```python
from build123d import *

# Parameters (mm, degrees)
F1_DEPTH = 325
F2_W     = 250
F2_H     = 650
F3_DEPTH = 900


with BuildPart() as f1:
    # F0 (on Right) → F1 (new body, symmetric)
    with BuildSketch(Plane.YZ):
        Polygon((100, 875.2594227621), (650.2305358614, 489.9838537988), (722.4783731793, 544.4265042209), (214.6667939321, 900), (100, 900), align=None)
        Polygon((650.2305358614, 489.9838537988), (0, 0), (150, 0), (727.9826985434, 435.5412033767), align=None)
        Polygon((722.4783731793, 544.4265042209), (650.2305358614, 489.9838537988), (727.9826985434, 435.5412033767), (800.2305358614, 489.9838537988), align=None)
        Polygon((1194.3403394584, 900), (722.4783731793, 544.4265042209), (800.2305358614, 489.9838537988), (1250, 828.9094551131), (1250, 900), align=None)
        Polygon((800.2305358614, 489.9838537988), (727.9826985434, 435.5412033767), (1350, 0), (1500, 0), align=None)
    extrude(amount=F1_DEPTH, both=True)

    # F2 (on Top) → F3 (cut, through all)
    with BuildSketch(Plane.XY):
        with Locations((200, 675)):
            Rectangle(F2_W, F2_H)
        with Locations((-200, 675)):
            Rectangle(F2_W, F2_H)
    extrude(amount=F3_DEPTH, mode=Mode.SUBTRACT)


solid = f1.part
```
CAD build for the part. Positions are in the model's coordinates, mm. A direction names the side the tool comes from. Coordinates: 2 decimals unless noted, no trailing zeros. Order: outer loops, then holes, each group sorted by start corner. A loop starts at its lowest first (then second) coordinate and runs counter-clockwise, first axis right, second up.
(1) Drill centre lines: L1, parallel to X at y = 965.5, z = 358.5; L2, parallel to Y at x = -25.5, z = 774; L3, parallel to Y at x = -10, z = 629.5. Where is each one in solid material? Low to high.
Solution:
L1: x = -75 to 75
L2: y = 244.61 to 394.61, 1027.13 to 1177.13
L3: y = 450.98 to 600.98, 835.37 to 985.37
(2) Pin check, flat tips, straight feed: pin 1 Ø1 at (x, z) = (-29, 332) entering from -Y; pin 2 Ø5 at (x, z) = (-88, 333) entering from -Y; pin 3 Ø1 at (x, z) = (88.5, 715.5) entering from +Y. Stop position of each tip, or through.
Solution:
pin 1: stops at y = 439.92
pin 2: stops at y = 1000
pin 3: stops at y = 1100.16
(3) Saw through at A-A, the plane x = -121. Write the cut outline in (y, z), and give its area (3 significant figures).
Solution:
outline: (0, 0) - (150, 0) - (350, 150.71) - (350, 263.74) - close; (100, 875.26) - (350, 700.21) - (350, 805.24) - (214.67, 900) - (100, 900) - close; (1000, 245.07) - (1350, 0) - (1500, 0) - (1000, 350.1) - close; (1000, 640.52) - (1250, 828.91) - (1250, 900) - (1194.34, 900) - (1000, 753.55) - close
area: 124,000 mm2
(4) Which spindle directions (+Z, -Z, +X, -X, +Y, -Y) get a long thin tool onto all of the face, cutting with end or side? Do faces 5 (the face through (4.55, 359.28, 798.74)), 6 (the face through (198, 350, 752)), 7 (the face through (-202, 1000, 696)), 8 (the face through (4.55, 1232.766, 187.119)). Say none if no direction does.
Solution:
face 5: +Z, +X, -X
face 6: +Z, -Z, +X
face 7: +Z, -Z, -X
face 8: +X, -X, +Y
(5) Saw through at B-B, the plane z = 221.5. Write the cut outline in (x, y), and give its area (3 significant figures).
Solution:
outline: (-325, 293.94) - (325, 293.94) - (325, 350) - (75, 350) - (75, 443.94) - (-75, 443.94) - (-75, 350) - (-325, 350) - close; (-325, 1033.67) - (325, 1033.67) - (325, 1183.67) - (-325, 1183.67) - close
area: 148,000 mm2
(6) Saw through at C-C, the plane y = 392. Write the cut outline in (x, z), and give its area (3 significant figures).
Solution:
outline: (-75, 182.36) - (75, 182.36) - (75, 295.39) - (-75, 295.39) - close; (-75, 670.8) - (75, 670.8) - (75, 775.83) - (-75, 775.83) - close
area: 32,700 mm2
(7) Saw through at D-D, the plane x = -22. Write the cut outline in (y, z), and give its area (3 significant figures).
Solution:
outline: (0, 0) - (150, 0) - (727.98, 435.54) - (1350, 0) - (1500, 0) - (800.23, 489.98) - (1250, 828.91) - (1250, 900) - (1194.34, 900) - (722.48, 544.43) - (214.67, 900) - (100, 900) - (100, 875.26) - (650.23, 489.98) - close
area: 258,000 mm2
(8) Mould opens along Z. For faces 1 (the face through (-325, 251, 824)), 2 (the face through (5, 74, 0)), 3 (the face through (4.55, 248.99, 770.935)), 4 (the face through (4.55, 1066.57, 803.72)) say: released by +Z, released by -Z, zero draft, split by the parting line, or undercut.
Solution:
face 1: zero draft
face 2: released by -Z
face 3: undercut
face 4: released by +Z
